Geometry: final body of the model. Coordinates: model frame, mm. A direction names the side the tool comes from. Give positions to 0.01 mm unless a question says otherwise; leave off trailing zeros. Write each loop counter-clockwise with the first axis right and the second up, starting at its lowest first coordinate (ties: lowest second). Pieces come first, ordered by that corner, then holes. Notation, with made-up numbers: M 65.5,11 L 70.5,11 A27 ccw 70.5,43 Z; hole C 24,-17 d1. An arc over 180 degrees is marked long. Use a Markdown table: item, result. Add a question column.
(1) Cut plane D-D (x = 16.17). Output: boundary loops of the cut face in (y, z).
(2) Material intervals for L1, parallel to X at y = 0.1, z = 1.6; L2, parallel to Y at x = 16.17, z = 0.4; L3, parallel to X at y = 0.95, z = 0.6, sorted ascending.
(3) Cut plane C-C (z = 1.5). Output: boundary loops of the cut face in (x, y).
(4) Pin query (flat end, axial travel): pin 1 Ø0.8 at (x, z) = (8.5, 1.5) entering from -Y; pin 2 Ø0.8 at (x, z) = (6, 1) entering from +Y; pin 3 Ø1.5 at (x, y) = (8.5, 1) entering from -Z. Return the tip coordinate at first contact, or that it passes through.
(5) Cut plane B-B (x = 0). Output: boundary loops of the cut face in (y, z), plus the area to 3 significant figures.
(6) Cut plane A-A (y = 0). Output: boundary loops of the cut face in (x, z).
(7) Reachability of faces 1 (the flat face through (8, 2.5, 1)), 2 (the flat face through (1.3, 0.7, -0.5)), 3 (the flat face through (8, -2.5, 1)) from +Z, -Z, +X, -X, +Y, -Y: full face, straight path, thin tool, end or side. Return the list, or none.
(8) Draft query along X for faces 4 (the flat face through (8, 0, 2.5)), 5 (the flat face through (8, 0, 0)). Return one class per face: released by +X, released by -X, zero draft, split by the parting line, or undercut.
```python
from build123d import *

# Parameters (mm, degrees)
SKETCH14_R          = 1.3
SKETCH14_R_2        = 1.2
BOSS_EXTRUDE1_DEPTH = 2.5
SKETCH15_R          = 3
SKETCH15_R_2        = 1.2
SKETCH15_R_3        = 1.3
BOSS_EXTRUDE2_DEPTH = 3


with BuildPart() as part:
    # Sketch14 → Boss-Extrude1 (new body)
    with BuildSketch(Plane.XY):
        with BuildLine():
            Line((16.17, 2.5), (0, 2.5))
            ThreePointArc((0, 2.5), (-2.5, 0), (0, -2.5))
            Line((0, -2.5), (16.17, -2.5))
            ThreePointArc((16.17, -2.5), (18.67, 0), (16.17, 2.5))
        make_face()
        Circle(SKETCH14_R, mode=Mode.SUBTRACT)
        with Locations((16.17, 0)):
            Circle(SKETCH14_R_2, mode=Mode.SUBTRACT)
    extrude(amount=BOSS_EXTRUDE1_DEPTH)

    # Sketch15 → Boss-Extrude2 (add)
    with BuildSketch(Plane.XY.offset(2.5)):
        with Locations((16.17, 0)):
            Circle(SKETCH15_R)
        with Locations((16.17, 0)):
            Circle(SKETCH15_R_2, mode=Mode.SUBTRACT)
        Circle(SKETCH15_R)
        Circle(SKETCH15_R_3, mode=Mode.SUBTRACT)
    extrude(amount=-BOSS_EXTRUDE2_DEPTH)


solid = part.part
```
Answer list:
| question | item | result |
|---|---|---|
| 1 | outline | M -3,-0.5 L -1.2,-0.5 L -1.2,2.5 L -3,2.5 Z; M 1.2,-0.5 L 3,-0.5 L 3,2.5 L 1.2,2.5 Z |
| 2 | L1 | -3 to -1.3, 1.3 to 14.97, 17.37 to 19.17 |
| 2 | L2 | -3 to -1.2, 1.2 to 3 |
| 2 | L3 | -2.85 to -0.89, 0.89 to 15.44, 16.9 to 19.02 |
| 3 | outline | M 1.66,-2.5 L 14.51,-2.5 A3 ccw long 14.51,2.5 L 1.66,2.5 A3 ccw long Z; hole C 0,0 d2.6; hole C 16.17,0 d2.4 |
| 4 | pin 1 | y = -2.5 |
| 4 | pin 2 | y = 2.5 |
| 4 | pin 3 | z = 0 |
| 5 | outline | M -3,-0.5 L -1.3,-0.5 L -1.3,2.5 L -3,2.5 Z; M 1.3,-0.5 L 3,-0.5 L 3,2.5 L 1.3,2.5 Z |
| 5 | area | 10.2 mm² |
| 6 | outline | M -3,-0.5 L -1.3,-0.5 L -1.3,2.5 L -3,2.5 Z; M 1.3,-0.5 L 3,-0.5 L 3,0 L 13.17,0 L 13.17,-0.5 L 14.97,-0.5 L 14.97,2.5 L 1.3,2.5 Z; M 17.37,-0.5 L 19.17,-0.5 L 19.17,2.5 L 17.37,2.5 Z |
| 7 | face 1 | +Z, -Z, +Y |
| 7 | face 2 | -Z, +X, -X, +Y, -Y |
| 7 | face 3 | +Z, -Z, -Y |
| 8 | face 4 | zero draft |
| 8 | face 5 | undercut |
